from build123d import *

# Parameters (mm, degrees)
CROQUIS2_R                = 4.25
SALIENTE_EXTRUIR1_DEPTH   = 15
SALIENTE_EXTRUIR1_2_DEPTH = 15
CROQUIS3_W                = 28.9
CROQUIS3_H                = 16
SALIENTE_EXTRUIR2_DEPTH   = 2


with BuildPart() as part:
    # Croquis2 → Saliente-Extruir1 (new body)
    with BuildSketch(Plane(origin=(0, 0, 0), x_dir=(0, 0, -1), z_dir=(1, 0, 0))):
        Circle(CROQUIS2_R)
    extrude(amount=SALIENTE_EXTRUIR1_DEPTH)



with BuildPart() as body_2:
    # Croquis2 → Saliente-Extruir1 2 (new body)
    with BuildSketch(Plane(origin=(0, 0, 0), x_dir=(0, 0, -1), z_dir=(1, 0, 0))):
        with BuildLine():
            Line((-14.45, 5), (-14.361406616, 5))
            ThreePointArc((-14.361406616, 5), (-9.765681466, 3.280086206), (-7.428313767, -1.034482759))
            ThreePointArc((-7.428313767, -1.034482759), (0, -7.5), (7.428313767, -1.034482759))
            ThreePointArc((7.428313767, -1.034482759), (9.765681466, 3.280086206), (14.361406616, 5))
            Line((14.361406616, 5), (14.45, 5))
            Line((14.45, 5), (14.45, -11))
            Line((14.45, -11), (-14.45, -11))
            Line((-14.45, -11), (-14.45, 5))
        make_face()
    extrude(amount=SALIENTE_EXTRUIR1_2_DEPTH)


with BuildPart() as part_1:
    add(part.part)

    add(body_2.part)  # Saliente-Extruir2 merges body 2
    # Croquis3 → Saliente-Extruir2 (add)
    with BuildSketch(Plane.ZY):
        with Locations((0, -3)):
            Rectangle(CROQUIS3_W, CROQUIS3_H)
    extrude(amount=-SALIENTE_EXTRUIR2_DEPTH)


solid = part_1.part
Here's how the part is built. I have some questions about the finished solid (model axes, mm). A direction names the side the tool comes from. Coordinates: 2 decimals unless noted, no trailing zeros. Order: outer loops, then holes, each group sorted by start corner. A loop starts at its lowest first (then second) coordinate and runs counter-clockwise, first axis right, second up. Notation, with made-up numbers: (-19.5, 64) - (13.5, 64) arc R21 cw to (13.5, 99) - close; hole circle Ø4 at (49, 81.25). An arc over 180 degrees is marked (long way). Use CSV: the item, a comma, the result in double quotes. Start each with the question number.
1. Suppose I cut it at B-B on z = 0. List the corners of the cut face in (x, y) for me.
2. Suppose I cut it at C-C on y = 3.5. List the corners of the cut face in (x, z) for me, then the cut area to 3 significant figures.
3. Suppose I cut it at A-A on x = 6.5. List the corners of the cut face in (y, z) for me, then the cut area to 3 significant figures.
4. If we mould it in two halves opening along Z, with no side actions, what happens to faces 4 (the face through (7, -3, 14.45)), 5 (the face through (7, -11, 0)), 6 (the face through (8.41, 3.23, -9.71))? For each: +Z half, -Z half, draft (parallel to the pull), parting line (faces both ways), or undercut.
5. Suppose I cut it at D-D on y = -6.25. List the corners of the cut face in (x, z) for me, then the cut area to 3 significant figures.
6. Please list where these lines run through material, in increasing order: line 1 (Y direction, x = 6.75, z = 0); line 2 (Z direction, x = 9, y = -3.25); line 3 (Z direction, x = 4.5, y = 1). Write a range as from..to.
7. For faces 1 (the face through (1, 5, 0)), 2 (the face through (8.409, 3.326, 9.819)), 3 (the face through (8.41, -7.5, 0.15)), which set-ups out of +Z, -Z, +X, -X, +Y, -Y let a thin tool reach every point of the face, with its end or its side?
Output:
1,outline,"(0, -11) - (15, -11) - (15, -7.5) - (2, -7.5) - (2, -4.25) - (15, -4.25) - (15, 4.25) - (2, 4.25) - (2, 5) - (0, 5) - close"
2,outline,"(0, -14.45) - (15, -14.45) - (15, -10.03) - (2, -10.03) - (2, -2.41) - (15, -2.41) - (15, 2.41) - (2, 2.41) - (2, 10.03) - (15, 10.03) - (15, 14.45) - (0, 14.45) - close"
2,area,"235 mm2"
3,outline,"(-11, -14.45) - (5, -14.45) - (5, -14.36) arc R7 ccw to (-1.03, -7.43) arc R7.5 cw to (-1.03, 7.43) arc R7 ccw to (5, 14.36) - (5, 14.45) - (-11, 14.45) - close; circle Ø8.5 at (0, 0)"
3,area,"336 mm2"
4,face 4,"+Z half"
4,face 5,"draft"
4,face 6,"undercut"
5,outline,"(0, -14.45) - (15, -14.45) - (15, -4.15) - (2, -4.15) - (2, 4.15) - (15, 4.15) - (15, 14.45) - (0, 14.45) - close"
5,area,"326 mm2"
6,line 1,"y = -11..-7.5, -4.25..4.25"
6,line 2,"z = -14.45..-6.76, -2.74..2.74, 6.76..14.45"
6,line 3,"z = -14.45..-8.04, -4.13..4.13, 8.04..14.45"
7,face 1,"+Z, -Z, +X, -X, +Y"
7,face 2,"+X, +Y"
7,face 3,"+X"
